from build123d import *

# Parameters (mm, degrees)
F0_W        = 5
F0_H        = 5
F1_DEPTH    = 20
F2_W        = 2.1819349527
F2_H        = 1.0583491623
F3_DEPTH    = 0.001
F5_DEPTH    = 5
F6_T1_DEPTH = 35
F6_T6_DEPTH = 35
F7_W        = 15
F7_H        = 3.1949503422
F8_DEPTH    = 5
F9_W        = 15
F9_H        = 3.1949481368
F10_DEPTH   = 5
F11_SIZE    = 4


# Not quite as in the source:
# - a fillet or chamfer that OpenCascade refuses, or shapes differently, is made with other operations: its cross-section is extruded or revolved along the edge and cut away or added


with BuildPart() as f1:
    # F0 (on Top) → F1 (new body)
    with BuildSketch(Plane.XY):
        with Locations((-70, -92)):
            Rectangle(F0_W, F0_H)
        with Locations((70, -92)):
            Rectangle(F0_W, F0_H)
        with BuildLine():
            Line((-67.5, -89.5), (-67.5, -26.4575131106))
            ThreePointArc((-67.5, -26.4575131106), (-71.2390342439, -13.4629120178), (-72.5, 0))
            Line((-72.5, 0), (-72.5, -89.5))
            Line((-72.5, -89.5), (-67.5, -89.5))
        make_face()
        with BuildLine():
            ThreePointArc((72.5, 0), (71.2390342439, -13.4629120178), (67.5, -26.4575131106))
            Line((67.5, -26.4575131106), (67.5, -89.5))
            Line((67.5, -89.5), (72.5, -89.5))
            Line((72.5, -89.5), (72.5, 0))
        make_face()
        with BuildLine():
            ThreePointArc((-67.5, 0), (0, 67.5), (67.5, 0))
            Line((67.5, 0), (67.5, -26.4575131106))
            ThreePointArc((67.5, -26.4575131106), (71.2390342439, -13.4629120178), (72.5, 0))
            ThreePointArc((72.5, 0), (0, 72.5), (-72.5, 0))
            ThreePointArc((-72.5, 0), (-71.2390342439, -13.4629120178), (-67.5, -26.4575131106))
            Line((-67.5, -26.4575131106), (-67.5, 0))
        make_face()
    extrude(amount=F1_DEPTH)

    # F2 (on face) → F3 (join)
    with BuildSketch(Plane(origin=(-72.5, 0, 0), x_dir=(0, -1, 0), z_dir=(-1, 0, 0))):
        with Locations((48.3409674764, 10.5291745812)):
            Rectangle(F2_W, F2_H)
    extrude(amount=F3_DEPTH)

    # F4 (on face) → F5 (join, symmetric)
    with BuildSketch(Plane(origin=(0, 0, 10), x_dir=(1, 0, 0), z_dir=(0, 0, -1))):
        Polygon((-67.5, 94.5), (-72.5, 94.5), (-77.5, 94.5), (-77.5, 88.8050496578), (-62.5, 88.8050496578), (-62.5, 94.5), align=None)
        Polygon((-77.5, 94.5), (-72.5, 94.5), (-67.5, 94.5), (-62.5, 94.5), (-62.5, 97), (-77.5, 97), align=None)
        Polygon((72.5142157078, 94.4999977946), (67.5142157078, 94.4999977946), (62.5142157078, 94.4999977946), (62.5142157078, 88.8050496578), (77.5142157078, 88.8050496578), (77.5142157078, 94.4999977946), align=None)
        Polygon((62.5142157078, 94.4999977946), (67.5142157078, 94.4999977946), (72.5142157078, 94.4999977946), (77.5142157078, 94.4999977946), (77.5142157078, 96.9999977946), (62.5142157078, 96.9999977946), align=None)
    extrude(amount=F5_DEPTH, both=True)

    # F6: fillet of radius 5 on 4 edges, made by hand

    # F6_s2 → F6_t1 (cut)
    with BuildSketch(Plane.XY.offset(-7.5)):
        with BuildLine():
            ThreePointArc((-77.5, -93.8050496578), (-76.0355339059, -90.2695157519), (-72.5, -88.8050496578))
            Line((-72.5, -88.8050496578), (-77.5, -88.8050496578))
            Line((-77.5, -88.8050496578), (-77.5, -93.8050496578))
        make_face()
        with BuildLine():
            ThreePointArc((72.5142157078, -88.8050496578), (76.0497496137, -90.2695157519), (77.5142157078, -93.8050496578))
            Line((77.5142157078, -93.8050496578), (77.5142157078, -88.8050496578))
            Line((77.5142157078, -88.8050496578), (72.5142157078, -88.8050496578))
        make_face()
        with BuildLine():
            ThreePointArc((-67.5, -88.8050496578), (-63.9644660941, -90.2695157519), (-62.5, -93.8050496578))
            Line((-62.5, -93.8050496578), (-62.5, -88.8050496578))
            Line((-62.5, -88.8050496578), (-67.5, -88.8050496578))
        make_face()
    extrude(amount=F6_T1_DEPTH, mode=Mode.SUBTRACT)


with BuildPart() as f6_tool4:
    # F6_s5 → F6_t6 (new body)
    with BuildSketch(Plane.XY.offset(-7.5)):
        with BuildLine():
            ThreePointArc((67.5142157078, -88.8050496578), (63.9786818018, -90.2695157519), (62.5142157078, -93.8050496578))
            Line((62.5142157078, -93.8050496578), (62.5142157078, -88.8050496578))
            Line((62.5142157078, -88.8050496578), (67.5142157078, -88.8050496578))
        make_face()
    extrude(amount=F6_T6_DEPTH)

    split(bisect_by=Plane.YZ.offset(67.5), keep=Keep.BOTTOM)


with BuildPart() as f1_1:
    add(f1.part)

    # F6_t3: cut F6_tool4
    add(f6_tool4.part, mode=Mode.SUBTRACT)

    # F7 (on face) → F8 (join)
    with BuildSketch(Plane.XY.offset(15)):
        with Locations((-70, -95.4025248289)):
            Rectangle(F7_W, F7_H)
    extrude(amount=F8_DEPTH)

    # F9 (on face) → F10 (join)
    with BuildSketch(Plane.XY.offset(15)):
        with Locations((70.0142157078, -95.4025237262)):
            Rectangle(F9_W, F9_H)
    extrude(amount=F10_DEPTH)

    # F11
    f11_edges = [f1_1.edges().sort_by_distance(p)[0] for p in [
        (-77.5, -95.402525, 20),
        (62.514216, -95.402524, 20),
        (-62.5, -95.402525, 20),
        (77.514216, -95.402524, 20),
    ]]
    chamfer(f11_edges, length=F11_SIZE)


solid = f1_1.part
Check sheet for the modelled part. Datum: model origin and axes. Units: mm. A direction names the side the tool comes from. Round coordinates to 2 decimals unless told otherwise and drop trailing zeros. Loops run counter-clockwise (first coordinate to the right, second up) from the corner with the lowest first, then second, coordinate; pieces in that order, holes last.
1. Sectioned sample at D-D on x = 44.5. Record the boundary of the cut face in (y, z).
2. Set-up check for faces 5 (the flat face through (-64.5, -95.4, 18)), 6 (the flat face through (66, -93.805, 17)), 7 (the flat face through (74, -93.805, 17)): record each of +Z, -Z, +X, -X, +Y, -Y from which the full face is reachable in a straight line by a thin tool's end or side.
3. Sectioned sample at C-C on y = 8.5. Record the boundary of the cut face in (x, z), and give its area (3 significant figures).
4. Sectioned sample at B-B on x = 0. Record the boundary of the cut face in (y, z), and give its area (3 significant figures).
5. Sectioned sample at A-A on y = -76. Record the boundary of the cut face in (x, z).
6. Mould release check, pull along X, two halves, no side actions. Record for faces 1 (the cylindrical face through (1.594, 72.482, 9.86)), 2 (the flat face through (-70, -94.5, 2)), 3 (the flat face through (66, -92, 15)), 4 (the cylindrical face through (-1.484, 67.484, 9.86)): released by +X, released by -X, zero draft, split by the parting line, or undercut.
7. Gauge pin test, flat ends, axial feed: pin 1 Ø10 at (y, z) = (-45.5, 7.5) entering from -X; pin 2 Ø1.5 at (x, z) = (69.5, 1.5) entering from -Y; pin 3 Ø4 at (y, z) = (-3.5, 2) entering from +X. Record the tip position at first contact, or that the pin passes through.
8. Scan lines: probe 1 along X at (y, z) = (-52, 13.25); probe 2 along X at (y, z) = (4.5, 3); probe 3 along Y at (x, z) = (-7.5, 8.75). Record each from-to range of solid material in increasing order.
Recorded:
1. outline: (50.75, 0) - (57.24, 0) - (57.24, 20) - (50.75, 20) - close
2. face 5: +Z, -Y
2. face 6: +Z
2. face 7: +Z, +X, +Y
3. outline: (-72, 0) - (-66.96, 0) - (-66.96, 20) - (-72, 20) - close; (66.96, 0) - (72, 0) - (72, 20) - (66.96, 20) - close
3. area: 201 mm2
4. outline: (67.5, 0) - (72.5, 0) - (72.5, 20) - (67.5, 20) - close
4. area: 100 mm2
5. outline: (-72.5, 0) - (-67.5, 0) - (-67.5, 20) - (-72.5, 20) - close; (67.5, 0) - (72.5, 0) - (72.5, 20) - (67.5, 20) - close
6. face 1: split by the parting line
6. face 2: zero draft
6. face 3: undercut
6. face 4: undercut
7. pin 1: stops at x = -72.5
7. pin 2: stops at y = -94.5
7. pin 3: stops at x = 72.5
8. probe 1: x = -72.5 to -67.5, 67.5 to 72.5
8. probe 2: x = -72.36 to -67.35, 67.35 to 72.36
8. probe 3: y = 67.08 to 72.11
